Can you work these out from the model? Positions are in its coordinate system, mm. Face numbers are marked on the shaded views. Round coordinates to 2 decimals unless told otherwise and drop trailing zeros. Loops run counter-clockwise (first coordinate to the right, second up) from the corner with the lowest first, then second, coordinate; pieces in that order, holes last.
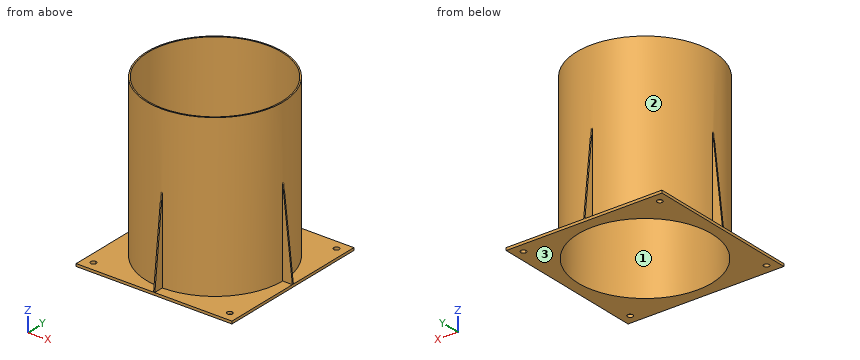
```python
from build123d import *

# Parameters (mm, degrees)
F0_W     = 120
F0_H     = 120
F0_R     = 51.5
F1_DEPTH = 2
F2_DEPTH = 125
F5_DEPTH = 0.5
F6_DEPTH = 0.5


with BuildPart() as f1:
    # F0 (on Top) → F1 (new body)
    with BuildSketch(Plane.XY):
        with Locations((0.0018474467, 3.25e-08)):
            Rectangle(F0_W, F0_H)
        with BuildLine():
            ThreePointArc((-52.4981525533, 50.4000000325), (-53.9830767937, 53.984924273), (-50.3981525533, 52.5000000325))
            Line((-50.3981525533, 52.5000000325), (0.0018477668, 52.5000000325))
            Line((0.0018477668, 52.5000000325), (50.4018474467, 52.5000000325))
            ThreePointArc((50.4018474467, 52.5000000325), (52.5018474467, 54.6000000325), (54.6018474467, 52.5000000325))
            ThreePointArc((54.6018474467, 52.5000000325), (53.9867716872, 51.015075792), (52.5018474467, 50.4000000325))
            Line((52.5018474467, 50.4000000325), (52.5018474467, 0))
            Line((52.5018474467, 0), (52.5018474467, -50.3999999675))
            ThreePointArc((52.5018474467, -50.3999999675), (53.9867716872, -51.015075727), (54.6018474467, -52.4999999675))
            ThreePointArc((54.6018474467, -52.4999999675), (52.5018474467, -54.5999999675), (50.4018474467, -52.4999999675))
            Line((50.4018474467, -52.4999999675), (0.0018474467, -52.4999999675))
            Line((0.0018474467, -52.4999999675), (-50.3981525533, -52.4999999675))
            ThreePointArc((-50.3981525533, -52.4999999675), (-53.9830767937, -53.984924208), (-52.4981525533, -50.3999999675))
            Line((-52.4981525533, -50.3999999675), (-52.4981525533, -3.4e-09))
            Line((-52.4981525533, -3.4e-09), (-52.4981525533, 50.4000000325))
        make_face(mode=Mode.SUBTRACT)
        with BuildLine():
            Line((0.0018477668, 52.5000000325), (-50.3981525533, 52.5000000325))
            ThreePointArc((-50.3981525533, 52.5000000325), (-51.0132283128, 51.015075792), (-52.4981525533, 50.4000000325))
            Line((-52.4981525533, 50.4000000325), (-52.4981525533, -3.4e-09))
            ThreePointArc((-52.4981525533, -3.4e-09), (-37.1212584536, 37.1231061243), (0.0018477668, 52.5))
        make_face()
        with BuildLine():
            Line((50.4018474467, 52.5000000325), (0.0018477668, 52.5000000325))
            ThreePointArc((0.0018477668, 52.5), (37.1249535722, 37.1231058991), (52.5018474467, 0))
            Line((52.5018474467, 0), (52.5018474467, 50.4000000325))
            ThreePointArc((52.5018474467, 50.4000000325), (51.0169232063, 51.015075792), (50.4018474467, 52.5000000325))
        make_face()
        with BuildLine():
            Line((52.5018474467, -50.3999999675), (52.5018474467, 0))
            ThreePointArc((52.5018474467, 0), (37.124953459, -37.1231060123), (0.0018474467, -52.5))
            Line((0.0018474467, -52.4999999675), (50.4018474467, -52.4999999675))
            ThreePointArc((50.4018474467, -52.4999999675), (51.0169232063, -51.015075727), (52.5018474467, -50.3999999675))
        make_face()
        with BuildLine():
            ThreePointArc((0.0018474467, -52.5), (-37.1212585644, -37.1231060135), (-52.4981525533, -3.4e-09))
            Line((-52.4981525533, -3.4e-09), (-52.4981525533, -50.3999999675))
            ThreePointArc((-52.4981525533, -50.3999999675), (-51.0132283128, -51.015075727), (-50.3981525533, -52.4999999675))
            Line((-50.3981525533, -52.4999999675), (0.0018474467, -52.4999999675))
        make_face()
        with BuildLine():
            ThreePointArc((52.5018474467, 0), (37.1249535722, 37.1231058991), (0.0018477668, 52.5))
            ThreePointArc((0.0018477668, 52.5), (-37.1212584536, 37.1231061243), (-52.4981525533, -3.4e-09))
            ThreePointArc((-52.4981525533, -3.4e-09), (-37.1212585644, -37.1231060135), (0.0018474467, -52.5))
            ThreePointArc((0.0018474467, -52.5), (37.124953459, -37.1231060123), (52.5018474467, 0))
        make_face()
        with Locations((0.0018474467, 0)):
            Circle(F0_R, mode=Mode.SUBTRACT)
    extrude(amount=F1_DEPTH)

    # F0 (on Top) → F2 (join)
    with BuildSketch(Plane.XY):
        with BuildLine():
            ThreePointArc((52.5018474467, 0), (37.1249535722, 37.1231058991), (0.0018477668, 52.5))
            ThreePointArc((0.0018477668, 52.5), (-37.1212584536, 37.1231061243), (-52.4981525533, -3.4e-09))
            ThreePointArc((-52.4981525533, -3.4e-09), (-37.1212585644, -37.1231060135), (0.0018474467, -52.5))
            ThreePointArc((0.0018474467, -52.5), (37.124953459, -37.1231060123), (52.5018474467, 0))
        make_face()
        with Locations((0.0018474467, 0)):
            Circle(F0_R, mode=Mode.SUBTRACT)
    extrude(amount=F2_DEPTH)

    # F3 (on Front) → F5 (join, symmetric)
    with BuildSketch(Plane.XZ):
        Polygon((-52.1482676268, 72.7708116174), (-59.9962957203, 2.0518270321), (-52.1482676268, 2.0518270321), align=None)
        Polygon((52.1482676268, 2.0518270321), (59.9962957203, 2.0518270321), (52.1482676268, 72.7708116174), align=None)
    extrude(amount=F5_DEPTH, both=True)

    # F4 (on Right) → F6 (join, symmetric)
    with BuildSketch(Plane.YZ):
        Polygon((-52.1623715758, 70.7189845853), (-60.0103996694, 0), (-52.1623715758, 0), align=None)
        Polygon((52.1341636777, 0), (59.9821917713, 0), (52.1341636777, 70.7189845853), align=None)
    extrude(amount=F6_DEPTH, both=True)


solid = f1.part
```
(1) For pin 1 (2 mm diameter, centred on x = 55, z = 32, fed in from +Y); pin 2 (1.5 mm diameter, centred on x = 20, z = 94.5, fed in from +Y); pin 3 (5 mm diameter, centred on y = 29, z = 87, fed in from +X), each with a flat end and sliding along its axis, tell me the tip position at first contact or that it passes through.
(2) Suppose I cut it at C-C (y = -21.5). Write out the boundary of the cut face in (x, z).
(3) We'd pull the mould along X, two halves only. Please class the marked faces 1, 2 and 3: released by +X, released by -X, zero draft, split by the parting line, or undercut.
(4) Suppose I cut it at B-B (z = 59.5). Write out the boundary of the cut face in (x, y), then the cut area to 3 significant figures.
(5) Suppose I cut it at A-A (x = -27). Write out the boundary of the cut face in (y, z), then the cut area to 3 significant figures.
(6) Suppose I cut it at D-D (z = 23). Write out the boundary of the cut face in (x, y), then the cut area to 3 significant figures.
(7) If I drill on line 1 (Y direction, x = -1, z = 63); line 2 (Z direction, x = -39, y = 49); line 3 (Y direction, x = 26.5, z = 89.5), over which ranges is the centre line in solid material (lowest first)?
Check result:
1. pin 1: stops at y = 0.5
1. pin 2: stops at y = 48.84
1. pin 3: stops at x = 45.32
2. outline: (-60, 0) - (-46.8, 0) - (-46.8, 125) - (-47.89, 125) - (-47.89, 2) - (-60, 2) - close; (46.8, 0) - (60, 0) - (60, 2) - (47.9, 2) - (47.9, 125) - (46.8, 125) - close
3. face 1: undercut
3. face 2: split by the parting line
3. face 3: zero draft
4. outline: (-53.62, -0.5) - (-52.5, -0.5) arc R52.5 ccw to (-0.5, -52.5) - (-0.5, -53.41) - (0.5, -53.41) - (0.5, -52.5) arc R52.5 ccw to (52.5, -0.5) - (53.62, -0.5) - (53.62, 0.5) - (52.5, 0.5) arc R52.5 ccw to (0.5, 52.5) - (0.5, 53.38) - (-0.5, 53.38) - (-0.5, 52.5) arc R52.5 ccw to (-52.5, 0.5) - (-53.62, 0.5) - close; hole circle Ø103 at (0, 0)
4. area: 331 mm2
5. outline: (-60, 0) - (-43.85, 0) - (-43.85, 125) - (-45.02, 125) - (-45.02, 2) - (-60, 2) - close; (43.85, 0) - (60, 0) - (60, 2) - (45.02, 2) - (45.02, 125) - (43.85, 125) - close
5. area: 352 mm2
6. outline: (-57.67, -0.5) - (-52.5, -0.5) arc R52.5 ccw to (-0.5, -52.5) - (-0.5, -57.46) - (0.5, -57.46) - (0.5, -52.5) arc R52.5 ccw to (52.5, -0.5) - (57.67, -0.5) - (57.67, 0.5) - (52.5, 0.5) arc R52.5 ccw to (0.5, 52.5) - (0.5, 57.43) - (-0.5, 57.43) - (-0.5, 52.5) arc R52.5 ccw to (-52.5, 0.5) - (-57.67, 0.5) - close; hole circle Ø103 at (0, 0)
6. area: 347 mm2
7. line 1: y = -52.49 to -51.49, 51.49 to 52.49
7. line 2: z = 0 to 2
7. line 3: y = -45.32 to -44.16, 44.16 to 45.32
